Read the model definition and answer for the solid it produces. Units are mm, in the model's axes. A direction names the side the tool comes from. Round coordinates to 2 decimals unless told otherwise and drop trailing zeros. Write each loop counter-clockwise with the first axis right and the second up, starting at its lowest first coordinate (ties: lowest second). Pieces come first, ordered by that corner, then holes. Notation, with made-up numbers: (-26.5, 39) - (27.5, 39) arc R14 ccw to (27.5, 49) - close; hole circle Ø9 at (44.25, -25). An arc over 180 degrees is marked (long way). Use one line per item in the form item = value. Start each with the question number.
1) Each of these flat-tipped pins is pushed along its axis until it touches: pin 1 (3 mm diameter, centred on x = -28.5, z = -4.5, fed in from -Y); pin 2 (10 mm diameter, centred on y = 6.5, z = 5.5, fed in from +X); pin 3 (3.5 mm diameter, centred on x = -19.5, z = -2.5, fed in from +Y); pin 4 (8 mm diameter, centred on x = 0, z = 22, fed in from -Y). Where does it stop, or does it pass through?
2) The part is cut by section B-B, the plane y = 19. Give the vertices of the cut face in (x, z).
3) The part is cut by section D-D, the plane z = 22. Give the vertices of the cut face in (x, y).
4) The part is cut by section C-C, the plane x = 0. Give the vertices of the cut face in (y, z), plus the area to 3 significant figures.
5) For faces 4 (the face through (28.73, 14.79, -20.63)), 5 (the face through (-38.927, 20, 0)), 6 (the face through (-31, 40, 0)), 7 (the face through (-19, 42, 6)), determine the directions among +Z, -Z, +X, -X, +Y, -Y from which every point of the face is accessible in a straight line to the end or side of a thin tool.
6) The part is cut by section A-A, the plane z = 0. Give the vertices of the cut face in (x, y).
7) Consider line 1 along X through (y, z) = (20.5, -0.5); line 2 along Z through (x, y) = (0, 40); line 3 along Y through (x, z) = (-24, -29). Determine where each line is inside the solid, lowest interval first. Write a range as from..to.
8) For a pull along X with two mould halves and no side action, classify faces 1 (the face through (-6.45, 29.01, 27.91)), 2 (the face through (-5.598, 20.706, -42.634)), 3 (the face through (-41, 40, 0)) as released by +X, released by -X, zero draft, split by the parting line, or undercut.
from build123d import *

# Parameters (mm, degrees)
SKETCH2_R           = 43
BOSS_EXTRUDE1_DEPTH = 42
SKETCH3_R           = 35.5
BOSS_EXTRUDE2_DEPTH = 2
CUT_EXTRUDE1_DEPTH  = 30
SKETCH6_W           = 12
SKETCH6_H           = 12
CUT_EXTRUDE2_DEPTH  = 3.5
SKETCH5_W           = 2
SKETCH5_H           = 10
CUT_EXTRUDE3_DEPTH  = 8
SKETCH7_R           = 6.75
CUT_EXTRUDE4_DEPTH  = 14
CUT_EXTRUDE5_DEPTH  = 2
CUT_EXTRUDE6_DEPTH  = 41
SKETCH10_W          = 10
SKETCH10_H          = 4
CUT_EXTRUDE7_DEPTH  = 10
SKETCH11_R          = 8.75
SKETCH11_R_2        = 6.75
BOSS_EXTRUDE3_DEPTH = 2


with BuildPart() as part:
    # Sketch2 → Boss-Extrude1 (new body)
    with BuildSketch(Plane(origin=(0, 0, 0), x_dir=(1, 0, 0), z_dir=(0, 1, 0))):
        Circle(SKETCH2_R)
    extrude(amount=BOSS_EXTRUDE1_DEPTH)

    # Sketch3 → Boss-Extrude2 (add)
    with BuildSketch(Plane(origin=(0, 42, 0), x_dir=(1, 0, 0), z_dir=(0, 1, 0))):
        Circle(SKETCH3_R)
    extrude(amount=BOSS_EXTRUDE2_DEPTH)

    # Sketch4 → Cut-Extrude1 (cut)
    with BuildSketch(Plane.XZ):
        with BuildLine():
            Line((-3.5, 32.813869019), (-3.5, 37.5))
            Line((-3.5, 37.5), (3.5, 37.5))
            Line((3.5, 37.5), (3.5, 32.813869019))
            ThreePointArc((3.5, 32.813869019), (28.578838325, 16.5), (30.167644167, -13.375845596))
            Line((30.167644167, -13.375845596), (34.225952642, -15.718911087))
            Line((34.225952642, -15.718911087), (30.725952642, -21.781088913))
            Line((30.725952642, -21.781088913), (26.667644167, -19.438023423))
            ThreePointArc((26.667644167, -19.438023423), (0, -33), (-26.667644167, -19.438023423))
            Line((-26.667644167, -19.438023423), (-30.725952642, -21.781088913))
            Line((-30.725952642, -21.781088913), (-34.225952642, -15.718911087))
            Line((-34.225952642, -15.718911087), (-30.167644167, -13.375845596))
            ThreePointArc((-30.167644167, -13.375845596), (-28.578838325, 16.5), (-3.5, 32.813869019))
        make_face()
    extrude(amount=-CUT_EXTRUDE1_DEPTH, mode=Mode.SUBTRACT)

    # Sketch6 → Cut-Extrude2 (cut)
    with BuildSketch(Plane(origin=(0, 44, 0), x_dir=(1, 0, 0), z_dir=(0, 1, 0))):
        with Locations((-19, 0)):
            Rectangle(SKETCH6_W, SKETCH6_H)
    extrude(amount=-CUT_EXTRUDE2_DEPTH, mode=Mode.SUBTRACT)

    # Sketch5 → Cut-Extrude3 (cut)
    with BuildSketch(Plane(origin=(0, 44, 0), x_dir=(1, 0, 0), z_dir=(0, 1, 0))):
        with Locations((-26, 0)):
            Rectangle(SKETCH5_W, SKETCH5_H)
    extrude(amount=-CUT_EXTRUDE3_DEPTH, mode=Mode.SUBTRACT)

    # Sketch7 → Cut-Extrude4 (cut)
    with BuildSketch(Plane(origin=(0, 44, 0), x_dir=(1, 0, 0), z_dir=(0, 1, 0))):
        with Locations((0, -22)):
            Circle(SKETCH7_R)
    extrude(amount=-CUT_EXTRUDE4_DEPTH, mode=Mode.SUBTRACT)

    # Sketch8 → Cut-Extrude5 (cut)
    with BuildSketch(Plane(origin=(0, 42, 0), x_dir=(1, 0, 0), z_dir=(0, 1, 0))):
        with BuildLine():
            Line((-42.708313008, 5), (-35.146123542, 5))
            ThreePointArc((-35.146123542, 5), (-35.5, 0), (-35.146123542, -5))
            Line((-35.146123542, -5), (-42.708313008, -5))
            ThreePointArc((-42.708313008, -5), (-43, 0), (-42.708313008, 5))
        make_face()
    extrude(amount=-CUT_EXTRUDE5_DEPTH, mode=Mode.SUBTRACT)

    # Sketch9 → Cut-Extrude6 (cut)
    with BuildSketch(Plane(origin=(0, 40, 0), x_dir=(1, 0, 0), z_dir=(0, 1, 0))):
        with BuildLine():
            Line((-35.146123542, 5), (-38.927218275, 5))
            Line((-38.927218275, 5), (-38.927218275, -5))
            Line((-38.927218275, -5), (-35.146123542, -5))
            ThreePointArc((-35.146123542, -5), (-35.5, 0), (-35.146123542, 5))
        make_face()
    extrude(amount=-CUT_EXTRUDE6_DEPTH, mode=Mode.SUBTRACT)

    # Sketch10 → Cut-Extrude7 (cut)
    with BuildSketch(Plane(origin=(-27, 0, 0), x_dir=(0, 0, -1), z_dir=(1, 0, 0))):
        with Locations((0, 38)):
            Rectangle(SKETCH10_W, SKETCH10_H)
    extrude(amount=-CUT_EXTRUDE7_DEPTH, mode=Mode.SUBTRACT)

    # Sketch11 → Boss-Extrude3 (add)
    with BuildSketch(Plane.XZ.offset(-30)):
        with Locations((0, 22)):
            Circle(SKETCH11_R)
        with Locations((0, 22)):
            Circle(SKETCH11_R_2, mode=Mode.SUBTRACT)
    extrude(amount=BOSS_EXTRUDE3_DEPTH)


solid = part.part
Geometry results:
q1.pin_1 = 30
q1.pin_2 = 43
q1.pin_3 = 40.5
q1.pin_4 = through
q2.outline = circle Ø86 at (0, 0); hole (-38.93, -5) - (-35.15, -5) arc R35.5 cw to (-35.15, 5) - (-38.93, 5) - close; hole (-34.23, -15.72) - (-30.73, -21.78) - (-26.67, -19.44) arc R33 ccw to (26.67, -19.44) - (30.73, -21.78) - (34.23, -15.72) - (30.17, -13.38) arc R33 ccw to (3.5, 32.81) - (3.5, 37.5) - (-3.5, 37.5) - (-3.5, 32.81) arc R33 ccw to (-30.17, -13.38) - close
q3.outline = (-36.95, 0) - (-24.6, 0) - (-24.6, 30) - (-8.75, 30) - (-8.75, 28) - (-6.75, 28) - (-6.75, 44) - (-27.86, 44) - (-27.86, 42) - (-36.95, 42) - close; (6.75, 28) - (8.75, 28) - (8.75, 30) - (24.6, 30) - (24.6, 0) - (36.95, 0) - (36.95, 42) - (27.86, 42) - (27.86, 44) - (6.75, 44) - close
q4.outline = (0, -43) - (42, -43) - (42, -35.5) - (44, -35.5) - (44, 15.25) - (28, 15.25) - (28, 13.25) - (30, 13.25) - (30, -33) - (0, -33) - close; (0, 37.5) - (30, 37.5) - (30, 30.75) - (28, 30.75) - (28, 28.75) - (44, 28.75) - (44, 35.5) - (42, 35.5) - (42, 43) - (0, 43) - close
q4.area = 1,460 mm2
q5.face_4 = -Y
q5.face_5 = +Y, -Y
q5.face_6 = none
q5.face_7 = +Y
q6.outline = (-43, 0) - (-38.93, 0) - (-38.93, 40) - (-43, 40) - close; (-35.5, 0) - (-33, 0) - (-33, 30) - (33, 30) - (33, 0) - (43, 0) - (43, 42) - (35.5, 42) - (35.5, 44) - (-13, 44) - (-13, 40.5) - (-25, 40.5) - (-25, 36) - (-35.5, 36) - close; (-35.5, 40) - (-27, 40) - (-27, 44) - (-35.5, 44) - close
q7.line_1 = -43..-38.93, -35.5..-33, 33..43
q7.line_2 = -43..15.25, 28.75..43
q7.line_3 = 0..42
q8.face_1 = undercut
q8.face_2 = split by the parting line
q8.face_3 = zero draft
